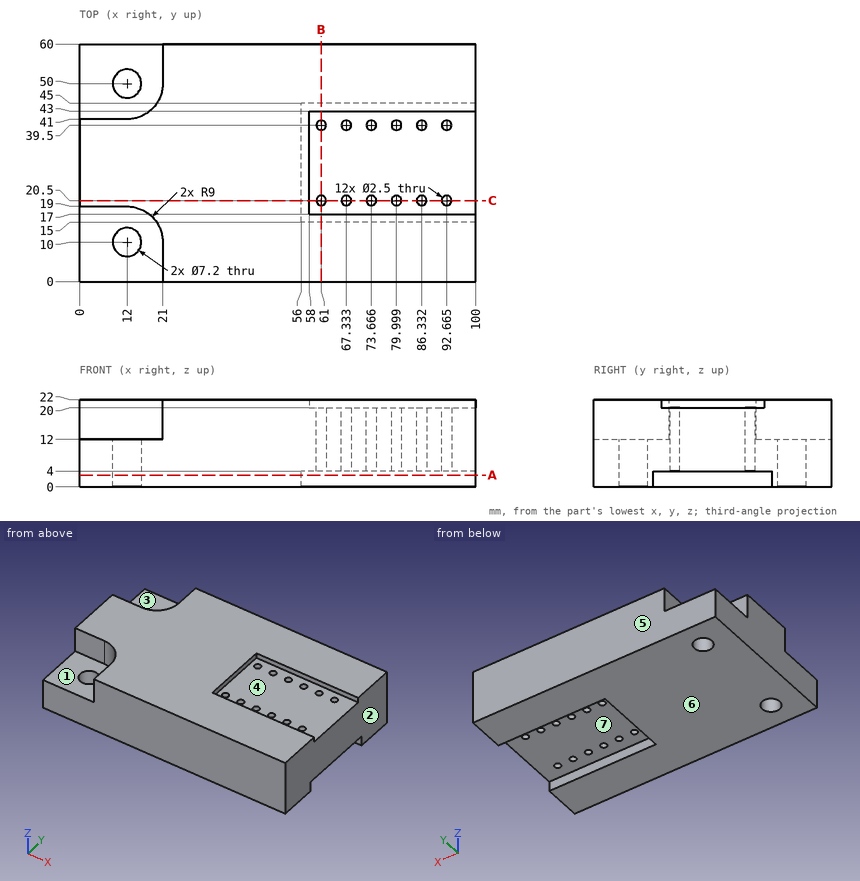
Design review of the part shown in the three views and the two pictorial views. Dimensions are in mm from the part's minimum x, y and z. A direction names the side the tool comes from. Round coordinates to 2 decimals unless told otherwise and drop trailing zeros. Loops run counter-clockwise (first coordinate to the right, second up) from the corner with the lowest first, then second, coordinate; pieces in that order, holes last. Notation, with made-up numbers: (-1, 42) - (22, 42) arc R25 ccw to (22, 64) - close; hole circle Ø2 at (51, 57). An arc over 180 degrees is marked (long way). One line per item, written item: value. Start each with the question number.
Item 1: Take a section at B-B (x = 61). Give the boundary of the cut face in (y, z), plus the area to 3 significant figures.
Item 2: The part is to be moulded in two halves that separate along Y. For the marked faces 4, 5, 6 and 7, say which applies: +Y half, -Y half, draft (parallel to the pull), parting line (faces both ways), or undercut.
Item 3: Clearance check with flat-ended pins moving along their axes: pin 1 Ø2 at (x, y) = (73.666, 20.5) entering from +Z; pin 2 Ø5.5 at (x, y) = (14, 5.5) entering from +Z; pin 3 Ø13 at (x, y) = (71.5, 34) entering from +Z; pin 4 Ø3 at (y, z) = (55, 16.5) entering from -X. State where each tip first meets the part, or that it passes through.
Item 4: Take a section at A-A (z = 3). Give the boundary of the cut face in (x, y), plus the area to 3 significant figures.
Item 5: For the marked faces 1, 2 and 3, list the 3-axis set-ups (+Z, -Z, +X, -X, +Y, -Y) from which the entire face can be reached by the end or side of a thin tool; tool diameter is ignored.
Item 6: For L1, parallel to Y at x = 12, z = 3.75; L2, parallel to Y at x = 13.5, z = 5.75; L3, parallel to Z at x = 18, y = 4, list the stretches that pass through material, from the lowest coordinate up.
Item 7: Take a section at C-C (y = 20.5). State how many separate pieces and enclosed holes the cut face has, plus the area to 3 significant figures.
Answer below:
1. outline: (0, 0) - (15, 0) - (15, 4) - (19.25, 4) - (19.25, 20) - (17, 20) - (17, 22) - (0, 22) - close; (21.75, 4) - (38.25, 4) - (38.25, 20) - (21.75, 20) - close; (40.75, 4) - (45, 4) - (45, 0) - (60, 0) - (60, 22) - (43, 22) - (43, 20) - (40.75, 20) - close
1. area: 1,070 mm2
2. face 4: undercut
2. face 5: +Y half
2. face 6: draft
2. face 7: undercut
3. pin 1: passes through
3. pin 2: stops at z = 12
3. pin 3: stops at z = 20
3. pin 4: stops at x = 21
4. outline: (0, 0) - (100, 0) - (100, 15) - (56, 15) - (56, 45) - (100, 45) - (100, 60) - (0, 60) - close; hole circle Ø7.2 at (12, 10); hole circle Ø7.2 at (12, 50)
4. area: 4,600 mm2
5. face 1: +Z, -X, -Y
5. face 2: +Z, -Z, +X, +Y, -Y
5. face 3: +Z, -X, +Y
6. L1: y = 0 to 6.4, 13.6 to 46.4, 53.6 to 60
6. L2: y = 0 to 6.73, 13.27 to 46.73, 53.27 to 60
6. L3: z = 0 to 12
7. separate pieces: 7
7. enclosed holes: 0
7. area: 1,700 mm2
